Could you check a few things on this model? Use its own coordinates, in mm. A direction names the side the tool comes from. Give positions to 0.01 mm unless a question says otherwise; leave off trailing zeros. Write each loop counter-clockwise with the first axis right and the second up, starting at its lowest first coordinate (ties: lowest second). Pieces come first, ordered by that corner, then holes. Notation, with made-up numbers: (14, 62.5) -> (46, 62.5) arc R21 ccw to (46, 99.5) -> close; hole circle Ø11 at (6.5, -12.5). An arc over 180 degrees is marked (long way). One line per question, with ' | ' between items.
Autodesk Inventor part; units mm, degrees
ref_plane "YZ Plane" through (0, 0, 0) normal (1, 0, 0) x (0, 1, 0)
ref_plane "XZ Plane" through (0, 0, 0) normal (0, 1, 0) x (-1, 0, 0)
ref_plane "XY Plane" through (0, 0, 0) normal (0, 0, 1) x (1, 0, 0)
sketch "Sketch1" plane through (0, 0, 0) normal (0, 0, 1) x (1, 0, 0)
  line L0 (-5.5, -15) -> (5.5, -15)
  line L1 (5.5, -15) -> (5.5, 15)
  line L2 (5.5, 15) -> (-5.5, 15)
  line L3 (-5.5, 15) -> (-5.5, -15)
  line L4 (-5.5, -15) -> (5.5, 15) construction
  line L5 (5.5, -15) -> (-5.5, 15) construction
  circle A0 centre (0, 0) radius 3
  circle A1 centre (0, 0) radius 3.7
  dimension "d0" = 5.5
  dimension "d1" = 15
extrude "Extrusion1" add sketch "Sketch1" along normal blind 2 contours L3 L2 L1 L0 | A0 | A1
sketch "Sketch2" plane through (0, 0, 0) normal (0, 0, -1) x (-1, 0, 0)
  line L0 (5.5, -15) -> (-5.5, -15)
  line L1 (5.5, 15) -> (5.5, -15)
  line L2 (-5.5, 15) -> (5.5, 15)
  line L3 (-5.5, -15) -> (-5.5, 15)
  circle A0 centre (0, 0) radius 4
extrude "Extrusion2" add sketch "Sketch2" along normal blind 4
sketch "Sketch3" plane through (0, 0, 2) normal (0, 0, 1) x (1, 0, 0)
  line L0 (-5.5, -15) -> (5.5, -15)
  line L1 (5.5, 15) -> (-5.5, 15)
  circle A0 centre (0, 10) radius 1.2
  circle A1 centre (0, -10) radius 1.2
  dimension "d6" = 2.4
  dimension "d7" = 2.4
  dimension "d8" = 5
  dimension "d9" = 5
extrude "Extrusion3" cut sketch "Sketch3" against normal blind 10
sketch "Sketch6" plane through (0, 0, -4) normal (0, 0, -1) x (-1, 0, 0)
  line L0 (-5.5, -15) -> (5.5, -15)
  line L1 (5.5, -15) -> (5.5, 15)
  line L2 (-5.5, 15) -> (-5.5, -15)
  line L3 (5.5, 12) -> (5.5, 13.2929)
  line L4 (5.5, -15) -> (5.5, -13.7071)
  line L5 (5.5, 12) -> (-5.5, 12)
  arc A0 (5, 5) -> (5.5, 3.882) centre (6.5, 5) ccw
  line L6 (5, 11.5) -> (5, 5)
  arc A1 (5.5, -12.3842) -> (5, -13.7071) centre (7, -13.7071) ccw
  line L7 (5, -13.7071) -> (5, -15)
  arc A2 (5.5, 12.618) -> (5, 11.5) centre (6.5, 11.5) ccw
  line L8 (5.5, 15) -> (-5.5, 15)
  dimension "d23" = 3
  dimension "d25" = 4
  dimension "d38" = 10
  dimension "d39" = 3.5
  dimension "d40" = 0.5
  dimension "d41" = 1.5
sketch "Sketch7" plane through (0, 0, -4) normal (0, 0, -1) x (-1, 0, 0)
  arc A0 (5.5, 12.8229) -> (5, 11.5) centre (7, 11.5) ccw
  line L0 (5.5, 15) -> (-5.5, 15)
  line L1 (-5.5, -15) -> (5.5, -15)
  line L2 (5.5, -15) -> (5.5, 15)
  line L3 (5, 5) -> (5, 11.5)
  line L4 (5, 11.5) -> (5, 15)
  arc A1 (5.5, -11.882) -> (5, -13) centre (6.5, -13) ccw
  line L5 (5, -13) -> (5, -15)
  line L6 (5, -15) -> (5.5, -15)
  line L7 (5.5, -15) -> (5.5, -11.882)
  line L8 (5.5, -15) -> (5.5, 15)
  line L9 (5, 15) -> (5.5, 15)
  line L10 (5.5, 15) -> (5.5, 12.8229)
  line L11 (5.5, 12.8229) -> (5.5, 11.5)
  line L12 (5.5, 11.5) -> (5.5, 10.597)
  line L13 (5.5, 10.597) -> (5, 10.597)
  line L14 (5, 10.597) -> (5, 11.5)
  point P0 (5.5, 3.6771)
  dimension "d29" = 3
  dimension "d30" = 2
  dimension "d51" = 0.5
extrude "Extrusion8" cut sketch "Sketch6" against normal blind 100 contours A2 L1 L5 | L5 L1 A0 L6 A2
extrude "Extrusion9" cut sketch "Sketch7" against normal blind 2.2
ref_plane "Work Plane1" through (0, -15, 2) normal (-1, 0, 0) x (0, 0, 1)
mirror "Mirror1" about plane through (0, -15, 2) normal (-1, 0, 0) of "Extrusion9", "Extrusion8"
sketch "Sketch8" plane through (0, 0, -4) normal (0, 0, -1) x (-1, 0, 0)
  circle A0 centre (0, 10) radius 1.2
  circle A1 centre (0, -10) radius 1.2
  circle A2 centre (0, 0) radius 4
  line L0 (-5, 15) -> (-5, 5)
  arc A3 (-5.5, 3.882) -> (-5, 5) centre (-6.5, 5) ccw
  line L1 (-5.5, 3.882) -> (-5.5, -11.882)
  arc A4 (-5, -13) -> (-5.5, -11.882) centre (-6.5, -13) ccw
  line L2 (-5, -13) -> (-5, -15)
  line L3 (-5, -15) -> (5, -15)
  line L4 (5, -15) -> (5, -13)
  arc A5 (5.5, -11.882) -> (5, -13) centre (6.5, -13) ccw
  line L5 (5.5, -11.882) -> (5.5, 3.882)
  arc A6 (5, 5) -> (5.5, 3.882) centre (6.5, 5) ccw
  line L6 (5, 5) -> (5, 15)
  line L7 (5, 15) -> (-5, 15)
extrude "Extrusion10" add sketch "Sketch8" along normal blind 0.2
sketch "Sketch9" plane through (0, 0, 0) normal (0, 0, -1) x (-1, 0, 0)
  circle A0 centre (0, 0) radius 4
  circle A1 centre (0, 0) radius 3
  dimension "d44" = 6
extrude "Extrusion11" cut sketch "Sketch9" against normal blind 100 contours A1
thread "Thread1"
thread "Thread2"
properties material "PAEK Plastic"
Q1. Imagine slicing it at A-A on z = -2.75. Please give me the cut outline in (x, y).
Answer below:
outline: (-5.5, -11.88) arc R1.5 cw to (-5, -13) -> (-5, -15) -> (5, -15) -> (5, -13) arc R1.5 cw to (5.5, -11.88) -> (5.5, 3.88) arc R1.5 cw to (5, 5) -> (5, 15) -> (-5, 15) -> (-5, 5) arc R1.5 cw to (-5.5, 3.88) -> close; hole circle Ø8 at (0, 0); hole circle Ø2.4 at (0, -10); hole circle Ø2.4 at (0, 10)
Q2. Imagine slicing it at B-B on y = 10. Please give me the cut outline in (x, z), and give its area (3 significant figures).
Answer below:
outline: (-5, -4.2) -> (-1.2, -4.2) -> (-1.2, 2) -> (-5, 2) -> close; (1.2, -4.2) -> (5, -4.2) -> (5, 2) -> (1.2, 2) -> close | area: 47.1 mm^2
Q3. Imagine slicing it at C-C on x = 0. Please give me the cut outline in (y, z), and give its area (3 significant figures).
Answer below:
outline: (-15, -4.2) -> (-11.2, -4.2) -> (-11.2, 2) -> (-15, 2) -> close; (-8.8, -4.2) -> (-4, -4.2) -> (-4, 0) -> (-3, 0) -> (-3, 2) -> (-8.8, 2) -> close; (3, 0) -> (4, 0) -> (4, -4.2) -> (8.8, -4.2) -> (8.8, 2) -> (3, 2) -> close; (11.2, -4.2) -> (15, -4.2) -> (15, 2) -> (11.2, 2) -> close | area: 111 mm^2
Q4. If I drill on line 1 along Y through (x, z) = (0, -2.25); line 2 along X through (y, z) = (-10, -0.5); line 3 along Y through (x, z) = (-1, -2.75), over which ranges is the centre line in solid material (lowest first)?
Answer below:
line 1: y = -15 to -11.2, -8.8 to -4, 4 to 8.8, 11.2 to 15 | line 2: x = -5.5 to -1.2, 1.2 to 5.5 | line 3: y = -15 to -10.66, -9.34 to -3.87, 3.87 to 9.34, 10.66 to 15
Q5. Will these pins go through, and if not, where does the flat tip stop? pin 1 (0.6 mm diameter, centred on y = -14, z = -2.5, fed in from +X); pin 2 (3 mm diameter, centred on y = 11, z = 0.5, fed in from -X); pin 3 (1.9 mm diameter, centred on x = 0, y = 10, fed in from +Z); pin 4 (1 mm diameter, centred on y = -13.5, z = -3, fed in from -X).
Answer below:
pin 1: stops at x = 5 | pin 2: stops at x = -5.38 | pin 3: passes through | pin 4: stops at x = -5
Q6. If we mould it in two halves opening along Y, with no side actions, what happens to faces 1 (the flat face through (0, -15, -1)), 2 (the cylindrical face through (0.079, -8.803, -1.057)), 3 (the cylindrical face through (0.079, 11.197, -1.057)), 4 (the flat face through (-5.5, 14, 0))? For each: +Y half, -Y half, draft (parallel to the pull), parting line (faces both ways), or undercut.
Answer below:
face 1: -Y half | face 2: undercut | face 3: undercut | face 4: draft
Q7. On a 3-axis mill with a long thin cutter (end or side, diameter ignored), from which of +Z, -Z, +X, -X, +Y, -Y can I reach the whole of each face in a straight line? I mean faces 5 (the flat face through (1, 3, 0)), 6 (the cylindrical face through (5.127, 12.104, 0.073)), 7 (the flat face through (5, -14, -3)). Say none if no direction works.
Answer below:
face 5: -Z | face 6: +Z, -Z, +X | face 7: -Z, +X, -Y
Q8. Imagine slicing it at D-D on y = 0. Please give me the cut outline in (x, z), and give its area (3 significant figures).
Answer below:
outline: (-5.5, -4.2) -> (-4, -4.2) -> (-4, 0) -> (-3, 0) -> (-3, 2) -> (-5.5, 2) -> close; (3, 0) -> (4, 0) -> (4, -4.2) -> (5.5, -4.2) -> (5.5, 2) -> (3, 2) -> close | area: 22.6 mm^2
